Verification items for the finished model (mm, model axes). A direction names the side the tool comes from. Coordinates: 2 decimals unless noted, no trailing zeros. Loops run counter-clockwise (first coordinate to the right, second up) from the corner with the lowest first, then second, coordinate; pieces in that order, holes last. Notation, with made-up numbers: (-7, 18) -> (18, 18) arc R21 ccw to (18, 35) -> close; hole circle Ø8 at (45.25, 55.5). An arc over 180 degrees is marked (long way). Answer as a JSON object with one key per item and string values. Group by question number.
Q1. Cross-section at B-B on y = 14.1. Record the boundary of the cut face in (x, z).
Q2. Cross-section at D-D on x = 36.4. Record the boundary of the cut face in (y, z).
Q3. Gauge pin test, flat ends, axial feed: pin 1 Ø4 at (x, y) = (100.5, 42.5) entering from -Z; pin 2 Ø4.5 at (x, y) = (85.5, 1.5) entering from -Z. Record the tip position at first contact, or that the pin passes through.
Q4. Release check for a two-part mould opening along Z. For faces 4 (the cylindrical face through (77.141, 35.403, 1.521)), 5 (the cylindrical face through (9.77, 76.23, -12.1)), 6 (the cylindrical face through (37.67, 2.03, -7.97)) record: released by +Z, released by -Z, zero draft, split by the parting line, or undercut.
Q5. Set-up check for faces 1 (the cylindrical face through (53.203, 57.059, 1.521)), 2 (the cylindrical face through (115.23, 2.03, -12.1)), 3 (the cylindrical face through (111.474, 2.028, -6.519)): record each of +Z, -Z, +X, -X, +Y, -Y from which the full face is reachable in a straight line by a thin tool's end or side.
Q6. Cross-section at A-A on z = -3.75. Record the boundary of the cut face in (x, y), and give its area (3 significant figures).
Q7. Scan lines: L1, parallel to Y at x = 100, z = -7; L2, parallel to X at y = 29, z = 1.75; L3, parallel to Y at x = 47, z = 1.85. Record each from-to range of solid material in increasing order.
Q8. Cross-section at C-C on x = 66. Record the boundary of the cut face in (y, z).
```python
from build123d import *

# Parameters (mm, degrees)
F0_W         = 125
F0_H         = 78.2
F1_DEPTH     = 3
F2_W         = 125
F2_H         = 4
F3_DEPTH     = 15
F5_D         = 3.2
F6_W         = 109
F6_H         = 4
F7_DEPTH     = 78.201
F9_D         = 3.2
F10_T1_DEPTH = 4
F10_T3_DEPTH = 4
F12_DEPTH    = 3


# Not quite as in the source:
# - a fillet or chamfer that OpenCascade refuses, or shapes differently, is made with other operations: its cross-section is extruded or revolved along the edge and cut away or added


with BuildPart() as f1:
    # F0 (on Top) → F1 (new body)
    with BuildSketch(Plane.XY):
        with Locations((62.5, 39.1)):
            Rectangle(F0_W, F0_H)
    extrude(amount=F1_DEPTH)

    # F2 (on face) → F3 (join)
    with BuildSketch(Plane(origin=(0, 0, 0), x_dir=(1, 0, 0), z_dir=(0, 0, -1))):
        with Locations((62.5, -76.2)):
            Rectangle(F2_W, F2_H)
        with Locations((62.5, -2)):
            Rectangle(F2_W, F2_H)
    extrude(amount=F3_DEPTH)

    # F5 (through all)
    with Locations(Plane.XZ):
        with Locations((113, -7), (36.4, -7)):
            Hole(F5_D / 2)

    # F6 (on face) → F7 (cut, through all)
    with BuildSketch(Plane.XZ):
        with Locations((62.5, -13)):
            Rectangle(F6_W, F6_H)
    extrude(amount=-F7_DEPTH, mode=Mode.SUBTRACT)

    # F9 (through all)
    with Locations(Plane.XY.offset(3)):
        with Locations((47, 14.1), (88, 14.1), (88, 64.1), (47, 64.1)):
            Hole(F9_D / 2)

    # F10: fillet of radius 5 on 4 edges, made by hand

    # F10_s2 → F10_t1 (join)
    with BuildSketch(Plane.XZ.offset(-4)):
        with BuildLine():
            ThreePointArc((112.1010205144, -11), (115.2632981746, -12.1270166538), (117, -15))
            Line((117, -15), (117, -11))
            Line((117, -11), (112.1010205144, -11))
        make_face()
        with BuildLine():
            ThreePointArc((8, -15), (9.7367018254, -12.1270166538), (12.8989794856, -11))
            Line((12.8989794856, -11), (8, -11))
            Line((8, -11), (8, -15))
        make_face()
    extrude(amount=F10_T1_DEPTH)

    # F10_s4 → F10_t3 (join)
    with BuildSketch(Plane.XZ.offset(-78.2)):
        with BuildLine():
            ThreePointArc((117, -15), (115.2632981746, -12.1270166538), (112.1010205144, -11))
            Line((112.1010205144, -11), (117, -11))
            Line((117, -11), (117, -15))
        make_face()
        with BuildLine():
            ThreePointArc((12.8989794856, -11), (9.7367018254, -12.1270166538), (8, -15))
            Line((8, -15), (8, -11))
            Line((8, -11), (12.8989794856, -11))
        make_face()
    extrude(amount=F10_T3_DEPTH)

    # F11 (on face) → F12 (cut, through all)
    with BuildSketch(Plane.XY.offset(3)):
        with BuildLine():
            Line((20, 58.2), (8, 58.2))
            ThreePointArc((8, 58.2), (5.1715728753, 57.0284271247), (4, 54.2))
            Line((4, 54.2), (4, 52.2))
            ThreePointArc((4, 52.2), (5.1715728753, 49.3715728753), (8, 48.2))
            Line((8, 48.2), (20, 48.2))
            ThreePointArc((20, 48.2), (22.8284271247, 49.3715728753), (24, 52.2))
            Line((24, 52.2), (24, 54.2))
            ThreePointArc((24, 54.2), (22.8284271247, 57.0284271247), (20, 58.2))
        make_face()
        with BuildLine():
            Line((20, 44.2), (8, 44.2))
            ThreePointArc((8, 44.2), (5.1715728753, 43.0284271247), (4, 40.2))
            Line((4, 40.2), (4, 38.2))
            ThreePointArc((4, 38.2), (5.1715728753, 35.3715728753), (8, 34.2))
            Line((8, 34.2), (20, 34.2))
            ThreePointArc((20, 34.2), (22.8284271247, 35.3715728753), (24, 38.2))
            Line((24, 38.2), (24, 40.2))
            ThreePointArc((24, 40.2), (22.8284271247, 43.0284271247), (20, 44.2))
        make_face()
        with BuildLine():
            Line((20, 30.2), (8, 30.2))
            ThreePointArc((8, 30.2), (5.1715728753, 29.0284271247), (4, 26.2))
            Line((4, 26.2), (4, 24.2))
            ThreePointArc((4, 24.2), (5.1715728753, 21.3715728753), (8, 20.2))
            Line((8, 20.2), (20, 20.2))
            ThreePointArc((20, 20.2), (22.8284271247, 21.3715728753), (24, 24.2))
            Line((24, 24.2), (24, 26.2))
            ThreePointArc((24, 26.2), (22.8284271247, 29.0284271247), (20, 30.2))
        make_face()
        with BuildLine():
            Line((44, 58.2), (32, 58.2))
            ThreePointArc((32, 58.2), (29.1715728753, 57.0284271247), (28, 54.2))
            Line((28, 54.2), (28, 52.2))
            ThreePointArc((28, 52.2), (29.1715728753, 49.3715728753), (32, 48.2))
            Line((32, 48.2), (44, 48.2))
            ThreePointArc((44, 48.2), (46.8284271247, 49.3715728753), (48, 52.2))
            Line((48, 52.2), (48, 54.2))
            ThreePointArc((48, 54.2), (46.8284271247, 57.0284271247), (44, 58.2))
        make_face()
        with BuildLine():
            Line((44, 44.2), (32, 44.2))
            ThreePointArc((32, 44.2), (29.1715728753, 43.0284271247), (28, 40.2))
            Line((28, 40.2), (28, 38.2))
            ThreePointArc((28, 38.2), (29.1715728753, 35.3715728753), (32, 34.2))
            Line((32, 34.2), (44, 34.2))
            ThreePointArc((44, 34.2), (46.8284271247, 35.3715728753), (48, 38.2))
            Line((48, 38.2), (48, 40.2))
            ThreePointArc((48, 40.2), (46.8284271247, 43.0284271247), (44, 44.2))
        make_face()
        with BuildLine():
            Line((44, 30.2), (32, 30.2))
            ThreePointArc((32, 30.2), (29.1715728753, 29.0284271247), (28, 26.2))
            Line((28, 26.2), (28, 24.2))
            ThreePointArc((28, 24.2), (29.1715728753, 21.3715728753), (32, 20.2))
            Line((32, 20.2), (44, 20.2))
            ThreePointArc((44, 20.2), (46.8284271247, 21.3715728753), (48, 24.2))
            Line((48, 24.2), (48, 26.2))
            ThreePointArc((48, 26.2), (46.8284271247, 29.0284271247), (44, 30.2))
        make_face()
        with BuildLine():
            Line((68, 58.2), (56, 58.2))
            ThreePointArc((56, 58.2), (53.1715728753, 57.0284271247), (52, 54.2))
            Line((52, 54.2), (52, 52.2))
            ThreePointArc((52, 52.2), (53.1715728753, 49.3715728753), (56, 48.2))
            Line((56, 48.2), (68, 48.2))
            ThreePointArc((68, 48.2), (70.8284271247, 49.3715728753), (72, 52.2))
            Line((72, 52.2), (72, 54.2))
            ThreePointArc((72, 54.2), (70.8284271247, 57.0284271247), (68, 58.2))
        make_face()
        with BuildLine():
            Line((68, 44.2), (56, 44.2))
            ThreePointArc((56, 44.2), (53.1715728753, 43.0284271247), (52, 40.2))
            Line((52, 40.2), (52, 38.2))
            ThreePointArc((52, 38.2), (53.1715728753, 35.3715728753), (56, 34.2))
            Line((56, 34.2), (68, 34.2))
            ThreePointArc((68, 34.2), (70.8284271247, 35.3715728753), (72, 38.2))
            Line((72, 38.2), (72, 40.2))
            ThreePointArc((72, 40.2), (70.8284271247, 43.0284271247), (68, 44.2))
        make_face()
        with BuildLine():
            Line((68, 30.2), (56, 30.2))
            ThreePointArc((56, 30.2), (53.1715728753, 29.0284271247), (52, 26.2))
            Line((52, 26.2), (52, 24.2))
            ThreePointArc((52, 24.2), (53.1715728753, 21.3715728753), (56, 20.2))
            Line((56, 20.2), (68, 20.2))
            ThreePointArc((68, 20.2), (70.8284271247, 21.3715728753), (72, 24.2))
            Line((72, 24.2), (72, 26.2))
            ThreePointArc((72, 26.2), (70.8284271247, 29.0284271247), (68, 30.2))
        make_face()
        with BuildLine():
            Line((92, 58.2), (80, 58.2))
            ThreePointArc((80, 58.2), (77.1715728753, 57.0284271247), (76, 54.2))
            Line((76, 54.2), (76, 52.2))
            ThreePointArc((76, 52.2), (77.1715728753, 49.3715728753), (80, 48.2))
            Line((80, 48.2), (92, 48.2))
            ThreePointArc((92, 48.2), (94.8284271247, 49.3715728753), (96, 52.2))
            Line((96, 52.2), (96, 54.2))
            ThreePointArc((96, 54.2), (94.8284271247, 57.0284271247), (92, 58.2))
        make_face()
        with BuildLine():
            Line((92, 44.2), (80, 44.2))
            ThreePointArc((80, 44.2), (77.1715728753, 43.0284271247), (76, 40.2))
            Line((76, 40.2), (76, 38.2))
            ThreePointArc((76, 38.2), (77.1715728753, 35.3715728753), (80, 34.2))
            Line((80, 34.2), (92, 34.2))
            ThreePointArc((92, 34.2), (94.8284271247, 35.3715728753), (96, 38.2))
            Line((96, 38.2), (96, 40.2))
            ThreePointArc((96, 40.2), (94.8284271247, 43.0284271247), (92, 44.2))
        make_face()
        with BuildLine():
            Line((92, 30.2), (80, 30.2))
            ThreePointArc((80, 30.2), (77.1715728753, 29.0284271247), (76, 26.2))
            Line((76, 26.2), (76, 24.2))
            ThreePointArc((76, 24.2), (77.1715728753, 21.3715728753), (80, 20.2))
            Line((80, 20.2), (92, 20.2))
            ThreePointArc((92, 20.2), (94.8284271247, 21.3715728753), (96, 24.2))
            Line((96, 24.2), (96, 26.2))
            ThreePointArc((96, 26.2), (94.8284271247, 29.0284271247), (92, 30.2))
        make_face()
        with BuildLine():
            Line((116, 58.2), (104, 58.2))
            ThreePointArc((104, 58.2), (101.1715728753, 57.0284271247), (100, 54.2))
            Line((100, 54.2), (100, 52.2))
            ThreePointArc((100, 52.2), (101.1715728753, 49.3715728753), (104, 48.2))
            Line((104, 48.2), (116, 48.2))
            ThreePointArc((116, 48.2), (118.8284271247, 49.3715728753), (120, 52.2))
            Line((120, 52.2), (120, 54.2))
            ThreePointArc((120, 54.2), (118.8284271247, 57.0284271247), (116, 58.2))
        make_face()
        with BuildLine():
            Line((116, 44.2), (104, 44.2))
            ThreePointArc((104, 44.2), (101.1715728753, 43.0284271247), (100, 40.2))
            Line((100, 40.2), (100, 38.2))
            ThreePointArc((100, 38.2), (101.1715728753, 35.3715728753), (104, 34.2))
            Line((104, 34.2), (116, 34.2))
            ThreePointArc((116, 34.2), (118.8284271247, 35.3715728753), (120, 38.2))
            Line((120, 38.2), (120, 40.2))
            ThreePointArc((120, 40.2), (118.8284271247, 43.0284271247), (116, 44.2))
        make_face()
        with BuildLine():
            Line((116, 30.2), (104, 30.2))
            ThreePointArc((104, 30.2), (101.1715728753, 29.0284271247), (100, 26.2))
            Line((100, 26.2), (100, 24.2))
            ThreePointArc((100, 24.2), (101.1715728753, 21.3715728753), (104, 20.2))
            Line((104, 20.2), (116, 20.2))
            ThreePointArc((116, 20.2), (118.8284271247, 21.3715728753), (120, 24.2))
            Line((120, 24.2), (120, 26.2))
            ThreePointArc((120, 26.2), (118.8284271247, 29.0284271247), (116, 30.2))
        make_face()
    extrude(amount=-F12_DEPTH, mode=Mode.SUBTRACT)


solid = f1.part
```
Computed values:
{
 "1": {"outline": "(0, 0) -> (45.4, 0) -> (45.4, 3) -> (0, 3) -> close; (48.6, 0) -> (86.4, 0) -> (86.4, 3) -> (48.6, 3) -> close; (89.6, 0) -> (125, 0) -> (125, 3) -> (89.6, 3) -> close"},
 "2": {"outline": "(0, -11) -> (4, -11) -> (4, -8.6) -> (0, -8.6) -> close; (0, -5.4) -> (4, -5.4) -> (4, 0) -> (20.2, 0) -> (20.2, 3) -> (0, 3) -> close; (30.2, 0) -> (34.2, 0) -> (34.2, 3) -> (30.2, 3) -> close; (44.2, 0) -> (48.2, 0) -> (48.2, 3) -> (44.2, 3) -> close; (58.2, 0) -> (74.2, 0) -> (74.2, -5.4) -> (78.2, -5.4) -> (78.2, 3) -> (58.2, 3) -> close; (74.2, -11) -> (78.2, -11) -> (78.2, -8.6) -> (74.2, -8.6) -> close"},
 "3": {"pin 1": "stops at z = 0", "pin 2": "stops at z = -11"},
 "4": {"face 4": "zero draft", "face 5": "released by -Z", "face 6": "undercut"},
 "5": {"face 1": "+Z, -Z", "face 2": "-Z, +Y, -Y", "face 3": "+Y, -Y"},
 "6": {"outline": "(0, 0) -> (125, 0) -> (125, 4) -> (0, 4) -> close; (0, 74.2) -> (125, 74.2) -> (125, 78.2) -> (0, 78.2) -> close", "area": "1,000 mm²"},
 "7": {"L1": "y = 0 to 4, 74.2 to 78.2", "L2": "x = 0 to 5.14, 22.86 to 29.14, 46.86 to 53.14, 70.86 to 77.14, 94.86 to 101.14, 118.86 to 125", "L3": "y = 0 to 12.5, 15.7 to 21.55, 28.85 to 35.55, 42.85 to 49.55, 56.85 to 62.5, 65.7 to 78.2"},
 "8": {"outline": "(0, -11) -> (4, -11) -> (4, 0) -> (20.2, 0) -> (20.2, 3) -> (0, 3) -> close; (30.2, 0) -> (34.2, 0) -> (34.2, 3) -> (30.2, 3) -> close; (44.2, 0) -> (48.2, 0) -> (48.2, 3) -> (44.2, 3) -> close; (58.2, 0) -> (74.2, 0) -> (74.2, -11) -> (78.2, -11) -> (78.2, 3) -> (58.2, 3) -> close"}
}
